Could you check a few things on this model? Use its own coordinates, in mm. Give positions to 0.01 mm unless a question says otherwise; leave off trailing zeros. Order: outer loops, then holes, each group sorted by start corner. A loop starts at its lowest first (then second) coordinate and runs counter-clockwise, first axis right, second up. Notation, with made-up numbers: (6.25, 60) -> (20.25, 60) arc R21 cw to (20.25, 74) -> close; hole circle Ø8 at (21, 65). An arc over 180 degrees is marked (long way). Write each question's results on one line, items separated by ' | '.
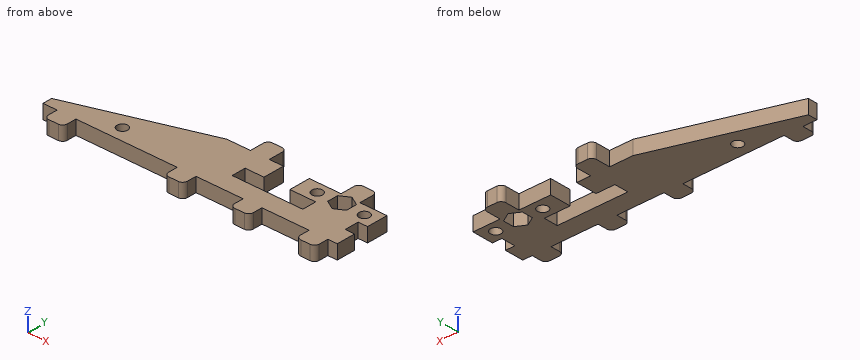
Autodesk Inventor part; units mm, degrees
ref_plane "YZ Plane" through (0, 0, 0) normal (1, 0, 0) x (0, 1, 0)
ref_plane "XZ Plane" through (0, 0, 0) normal (0, 1, 0) x (-1, 0, 0)
ref_plane "XY Plane" through (0, 0, 0) normal (0, 0, 1) x (1, 0, 0)
sketch "Sketch1" plane through (0, 0, 0) normal (0, 0, 1) x (1, 0, 0)
  line L0 (0, 4) -> (0, 0)
  line L1 (0, 0) -> (125, 0)
  line L2 (0, 4) -> (57, 23)
  line L3 (103, 14) -> (103, 8)
  line L4 (103, 8) -> (73, 8)
  line L5 (73, 8) -> (73, 14)
  line L6 (125, 14) -> (121, 14)
  line L7 (121, 14) -> (121, 8)
  line L8 (121, 8) -> (125, 8)
  line L9 (125, 0) -> (125, 8)
  line L10 (125, 14) -> (125, 23)
  line L11 (81, 23) -> (81, 14)
  line L12 (92, 14) -> (92, 23)
  line L13 (73, 14) -> (81, 14)
  line L14 (92, 14) -> (103, 14)
  line L15 (81, 14) -> (92, 14) construction
  circle A0 centre (86.5, 19.099) radius 7.5 construction
  circle A1 centre (86.5, 19.099) radius 4 construction
  line L16 (113.5, 21.4084) -> (113.5, 16.7896)
  line L17 (113.5, 16.7896) -> (109.5, 14.4802)
  line L18 (109.5, 14.4802) -> (105.5, 16.7896)
  line L19 (105.5, 16.7896) -> (105.5, 21.4084)
  line L20 (105.5, 21.4084) -> (109.5, 23.7178)
  line L21 (109.5, 23.7178) -> (113.5, 21.4084)
  circle A2 centre (109.5, 19.099) radius 2.5 construction
  line L22 (105.5, 23) -> (105.5, 29)
  line L23 (107.5, 31) -> (111.5, 31)
  line L24 (113.5, 29) -> (113.5, 23)
  arc A3 (107.5, 31) -> (105.5, 29) centre (107.5, 29) ccw
  arc A4 (113.5, 29) -> (111.5, 31) centre (111.5, 29) ccw
  line L25 (125, 23) -> (113.5, 23)
  line L26 (105.5, 23) -> (92, 23)
  circle A5 centre (99.5, 18.5) radius 4.5 construction
  circle A6 centre (119.5, 18.5) radius 4.5 construction
  circle A7 centre (99.5, 18.5) radius 2.25
  circle A8 centre (119.5, 18.5) radius 2.25
  line L27 (67, 23) -> (67, 29)
  line L28 (69, 31) -> (73, 31)
  line L29 (75, 29) -> (75, 23)
  arc A9 (69, 31) -> (67, 29) centre (69, 29) ccw
  arc A10 (75, 29) -> (73, 31) centre (73, 29) ccw
  line L30 (81, 23) -> (75, 23)
  line L31 (67, 23) -> (57, 23)
  point P0 (81, 14)
  point P1 (92, 14)
  point P2 (86.5, 14)
  point P3 (125, 18.5)
  point P4 (109.5, 31)
  dimension "d0" = 8
  dimension "d2" = 6
  dimension "d3" = 4
  dimension "d4" = 15
  dimension "d5" = 8
  dimension "d6" = 9
  dimension "d7" = 11
  dimension "d8" = 11
  dimension "d9" = 8
  dimension "d10" = 5
  dimension "d11" = 2
  dimension "d12" = 8
  dimension "d13" = 9
  dimension "d14" = 9
  dimension "d15" = 10
  dimension "d16" = 10
  dimension "d17" = 4.5
  dimension "d18" = 4.5
  dimension "d19" = 13
  dimension "d20" = 5.5
  dimension "d21" = 18
  dimension "d22" = 2
  dimension "d23" = 8
  dimension "d24" = 6
  dimension "d25" = 10
  dimension "d27" = 30
  dimension "d28" = 4
  dimension "d30" = 8
  dimension "d31" = 125
extrude "Extrusion1" add sketch "Sketch1" along normal blind 6
sketch "Sketch2" plane through (0, 0, 6) normal (0, 0, 1) x (1, 0, 0)
  line L0 (0, 4) -> (0, 0)
  line L1 (0, 0) -> (125, 0)
  line L2 (6, 0) -> (14, 0)
  line L3 (14, 0) -> (14, -4)
  line L4 (12, -6) -> (8, -6)
  line L5 (6, -4) -> (6, 0)
  line L6 (57, 0) -> (65, 0)
  line L7 (65, 0) -> (65, -4)
  line L8 (63, -6) -> (59, -6)
  line L9 (57, -4) -> (57, 0)
  line L10 (85, 0) -> (93, 0)
  line L11 (93, 0) -> (93, -4)
  line L12 (91, -6) -> (87, -6)
  line L13 (85, -4) -> (85, 0)
  line L14 (113, 0) -> (121, 0)
  line L15 (121, 0) -> (121, -4)
  line L16 (119, -6) -> (115, -6)
  line L17 (113, -4) -> (113, 0)
  arc A0 (6, -4) -> (8, -6) centre (8, -4) ccw
  arc A1 (12, -6) -> (14, -4) centre (12, -4) ccw
  arc A2 (57, -4) -> (59, -6) centre (59, -4) ccw
  arc A3 (63, -6) -> (65, -4) centre (63, -4) ccw
  arc A4 (85, -4) -> (87, -6) centre (87, -4) ccw
  arc A5 (91, -6) -> (93, -4) centre (91, -4) ccw
  arc A6 (113, -4) -> (115, -6) centre (115, -4) ccw
  arc A7 (119, -6) -> (121, -4) centre (119, -4) ccw
  dimension "d34" = 2
  dimension "d35" = 8
  dimension "d36" = 8
  dimension "d37" = 8
  dimension "d38" = 8
  dimension "d39" = 6
  dimension "d40" = 6
  dimension "d41" = 43
  dimension "d42" = 20
  dimension "d43" = 20
extrude "Extrusion2" add sketch "Sketch2" against normal blind 6
sketch "Sketch3" plane through (0, 0, 6) normal (0, 0, 1) x (1, 0, 0)
  line L0 (0, 4) -> (0, 0)
  line L1 (14, 0) -> (57, 0)
  circle A0 centre (28.2, 6) radius 2.25
  circle A1 centre (28.2, 6) radius 4.5 construction
  dimension "d46" = 4.5
  dimension "d47" = 6
  dimension "d48" = 28.2
  dimension "d51" = 9
extrude "Extrusion3" cut sketch "Sketch3" against normal through all
properties part number "x_motor_wall_upper"
Q1. I need wall thicknesses on line 1 along X through (y, z) = (-4, 3.15); line 2 along Y through (x, z) = (99.5, 2.1); line 3 along X through (y, z) = (29, 1.85). Which ranges of each line are inside material? Lowest first, please.
Here are the results:
line 1: x = 6 to 14, 57 to 65, 85 to 93, 113 to 121 | line 2: y = 0 to 8, 14 to 16.25, 20.75 to 23 | line 3: x = 67 to 75, 105.5 to 113.5
Q2. Suppose I cut it at A-A on y = 6. Please give me the cut outline in (x, z).
Here are the results:
outline: (6, 0) -> (25.95, 0) -> (25.95, 6) -> (6, 6) -> close; (30.45, 0) -> (125, 0) -> (125, 6) -> (30.45, 6) -> close
Q3. I'm going to push flat-ended pins straight in: pin 1 Ø6 at (x, y) = (28.2, 6) entering from -Z; pin 2 Ø3 at (y, z) = (10, 3.5) entering from +X; pin 3 Ø1.8 at (x, z) = (64, 4.5) entering from +Y; pin 4 Ø3 at (y, z) = (-3, 3) entering from -X. Where does each tip first touch, or does it pass through?
Here are the results:
pin 1: stops at z = 0 | pin 2: stops at x = 121 | pin 3: stops at y = 23 | pin 4: stops at x = 6
Q4. Suppose I cut it at C-C on y = 18.5. Please give me the cut outline in (x, z), and give its area (3 significant figures).
Here are the results:
outline: (43.5, 0) -> (81, 0) -> (81, 6) -> (43.5, 6) -> close; (92, 0) -> (97.25, 0) -> (97.25, 6) -> (92, 6) -> close; (101.75, 0) -> (105.5, 0) -> (105.5, 6) -> (101.75, 6) -> close; (113.5, 0) -> (117.25, 0) -> (117.25, 6) -> (113.5, 6) -> close; (121.75, 0) -> (125, 0) -> (125, 6) -> (121.75, 6) -> close | area: 321 mm²
Q5. Suppose I cut it at D-D on x = 99.5. Please give me the cut outline in (y, z).
Here are the results:
outline: (0, 0) -> (8, 0) -> (8, 6) -> (0, 6) -> close; (14, 0) -> (16.25, 0) -> (16.25, 6) -> (14, 6) -> close; (20.75, 0) -> (23, 0) -> (23, 6) -> (20.75, 6) -> close
Q6. Suppose I cut it at B-B on x = 28.2. Please give me the cut outline in (y, z).
Here are the results:
outline: (0, 0) -> (3.75, 0) -> (3.75, 6) -> (0, 6) -> close; (8.25, 0) -> (13.4, 0) -> (13.4, 6) -> (8.25, 6) -> close
